```python
from build123d import *

# Parameters (mm, degrees)
SKETCH_1_R             = 7
EXTRUDE_1_DEPTH        = 160
EXTRUDE_1_DEPTH_BACK   = 36
SKETCH_2_R             = 7
EXTRUDE_2_DEPTH        = 8
SKETCH_3_W             = 18
SKETCH_3_H             = 11
EXTRUDE_3_DEPTH        = 15
EXTRUDE_4_DEPTH        = 30
SKETCH_5_W             = 60
SKETCH_5_H             = 40
EXTRUDE_5_DEPTH        = 6
SKETCH_6_W             = 60
SKETCH_6_H             = 6
EXTRUDE_6_DEPTH        = 60
SKETCH_7_W             = 29.455878384
SKETCH_7_H             = 4
EXTRUDE_7_DEPTH        = 8
PATTERN_LINEAR_1_COUNT = 2
PATTERN_LINEAR_1_PITCH = 52
SKETCH_8_W             = 118.40385017
SKETCH_8_H             = 95.184754192
CUT_EXTRUDE_1_DEPTH    = 200


with BuildPart() as part:
    # 草图1 → 凸台-拉伸1 (new body, two sides)
    with BuildSketch(Plane.XY) as extrude_1_sk:
        Circle(SKETCH_1_R)
    extrude(amount=EXTRUDE_1_DEPTH)
    extrude(extrude_1_sk.sketch, amount=-EXTRUDE_1_DEPTH_BACK)

    # 草图2 → 凸台-拉伸2 (add)
    with BuildSketch(Plane(origin=(0, 0, -36), x_dir=(-1, 0, 0), z_dir=(0, 0, -1))):
        Polygon((20, 7.5), (15, 12.5), (-15, 12.5), (-20, 7.5), (-20, -7.5), (-15, -12.5), (15, -12.5), (20, -7.5), align=None)
        Circle(SKETCH_2_R, mode=Mode.SUBTRACT)
        Circle(SKETCH_2_R)
    extrude(amount=EXTRUDE_2_DEPTH)

    # 草图3 → 凸台-拉伸3 (add)
    with BuildSketch(Plane(origin=(0, 0, -44), x_dir=(-1, 0, 0), z_dir=(0, 0, -1))):
        Rectangle(SKETCH_3_W, SKETCH_3_H)
    extrude(amount=EXTRUDE_3_DEPTH)

    # 草图4 → 凸台-拉伸4 (add)
    with BuildSketch(Plane(origin=(0, 0, -59), x_dir=(-1, 0, 0), z_dir=(0, 0, -1))):
        with BuildLine():
            Line((-15, -12.5), (-15, 12.5))
            ThreePointArc((-15, 12.5), (-27.5, 0), (-15, -12.5))
        make_face()
        with BuildLine():
            ThreePointArc((-3.77502784, 5.5), (-8.385621722, 10.606601718), (-15, 12.5))
            Line((-15, 12.5), (-15, -12.5))
            ThreePointArc((-15, -12.5), (-8.385621722, -10.606601718), (-3.77502784, -5.5))
            Line((-3.77502784, -5.5), (-9, -5.5))
            Line((-9, -5.5), (-9, 5.5))
            Line((-9, 5.5), (-3.77502784, 5.5))
        make_face()
        with BuildLine():
            ThreePointArc((-2.5, 0), (-2.822928267, 2.822928267), (-3.77502784, 5.5))
            Line((-3.77502784, 5.5), (-9, 5.5))
            Line((-9, 5.5), (-9, -5.5))
            Line((-9, -5.5), (-3.77502784, -5.5))
            ThreePointArc((-3.77502784, -5.5), (-2.822928267, -2.822928267), (-2.5, 0))
        make_face()
        with BuildLine():
            ThreePointArc((3.77502784, -5.5), (2.5, 0), (3.77502784, 5.5))
            Line((3.77502784, 5.5), (-3.77502784, 5.5))
            ThreePointArc((-3.77502784, 5.5), (-2.822928267, 2.822928267), (-2.5, 0))
            ThreePointArc((-2.5, 0), (-2.822928267, -2.822928267), (-3.77502784, -5.5))
            Line((-3.77502784, -5.5), (3.77502784, -5.5))
        make_face()
        with BuildLine():
            Line((9, 5.5), (3.77502784, 5.5))
            ThreePointArc((3.77502784, 5.5), (2.5, 0), (3.77502784, -5.5))
            Line((3.77502784, -5.5), (9, -5.5))
            Line((9, -5.5), (9, 5.5))
        make_face()
        with BuildLine():
            Line((15, -12.5), (15, 12.5))
            ThreePointArc((15, 12.5), (8.385621722, 10.606601718), (3.77502784, 5.5))
            Line((3.77502784, 5.5), (9, 5.5))
            Line((9, 5.5), (9, -5.5))
            Line((9, -5.5), (3.77502784, -5.5))
            ThreePointArc((3.77502784, -5.5), (8.385621722, -10.606601718), (15, -12.5))
        make_face()
        with BuildLine():
            ThreePointArc((27.5, 0), (23.838834765, 8.838834765), (15, 12.5))
            Line((15, 12.5), (15, -12.5))
            ThreePointArc((15, -12.5), (23.838834765, -8.838834765), (27.5, 0))
        make_face()
        with BuildLine():
            Line((-15, -12.5), (15, -12.5))
            ThreePointArc((15, -12.5), (8.385621722, -10.606601718), (3.77502784, -5.5))
            Line((3.77502784, -5.5), (-3.77502784, -5.5))
            ThreePointArc((-3.77502784, -5.5), (-8.385621722, -10.606601718), (-15, -12.5))
        make_face()
        with BuildLine():
            ThreePointArc((3.77502784, 5.5), (8.385621722, 10.606601718), (15, 12.5))
            Line((15, 12.5), (-15, 12.5))
            ThreePointArc((-15, 12.5), (-8.385621722, 10.606601718), (-3.77502784, 5.5))
            Line((-3.77502784, 5.5), (3.77502784, 5.5))
        make_face()
    extrude(amount=EXTRUDE_4_DEPTH)

    # 草图5 → 凸台-拉伸5 (add)
    with BuildSketch(Plane(origin=(0, 0, -89), x_dir=(-1, 0, 0), z_dir=(0, 0, -1))):
        Rectangle(SKETCH_5_W, SKETCH_5_H)
    extrude(amount=EXTRUDE_5_DEPTH)

    # 草图6 → 凸台-拉伸6 (add)
    with BuildSketch(Plane(origin=(0, 0, -95), x_dir=(-1, 0, 0), z_dir=(0, 0, -1))):
        with Locations((0, 17)):
            Rectangle(SKETCH_6_W, SKETCH_6_H)
        with Locations((0, -17)):
            Rectangle(SKETCH_6_W, SKETCH_6_H)
    extrude(amount=EXTRUDE_6_DEPTH)

    # 草图7 → 凸台-拉伸7 (add)
    with BuildSketch(Plane.ZY.offset(30)):
        Polygon((-125, 8), (-125, 14), (-155, 14), (-160, 14), (-160, 8), align=None)
        Polygon((-125, -8), (-160, -8), (-160, -14), (-155, -14), (-125, -14), align=None)
        Polygon((-160, 8), (-160, 14), (-166, 14), (-166, 4), (-166, 0), (-166, -4), (-166, -14), (-160, -14), (-160, -8), align=None)
        with Locations((-180.727939192, -2)):
            Rectangle(SKETCH_7_W, SKETCH_7_H)
        with Locations((-180.727939192, 2)):
            Rectangle(SKETCH_7_W, SKETCH_7_H)
    extrude_7 = extrude(amount=-EXTRUDE_7_DEPTH)

    # 阵列(线性)1: 凸台-拉伸7 ×2
    with Locations(*[(i * PATTERN_LINEAR_1_PITCH, 0, 0) for i in range(1, PATTERN_LINEAR_1_COUNT)]):
        add(extrude_7)

    # 草图8 → 切除-拉伸1 (cut)
    with BuildSketch(Plane.XY.offset(-59)):
        Rectangle(SKETCH_8_W, SKETCH_8_H)
    extrude(amount=-CUT_EXTRUDE_1_DEPTH, mode=Mode.SUBTRACT)


solid = part.part
```
Check sheet for the modelled part. Datum: model origin and axes. Units: mm. A direction names the side the tool comes from. Coordinates: 2 decimals unless noted, no trailing zeros. Write each loop counter-clockwise with the first axis right and the second up, starting at its lowest first coordinate (ties: lowest second). Pieces come first, ordered by that corner, then holes. Notation, with made-up numbers: (41, 56.25) -> (72, 56.25) arc R16 cw to (72, 83.25) -> close; hole circle Ø8 at (-10, 36). An arc over 180 degrees is marked (long way). Use a Markdown table: item, result.
1. Sectioned sample at D-D (y = -9.5). Enter the section's corners in (x, z).
Reported:
| item | result |
|---|---|
| outline | (-18, -44) -> (18, -44) -> (18, -36) -> (-18, -36) -> close |
2. Tool access check on faces 1 (the flat face through (0, -5.5, -51)), 2 (the flat face through (0, 5.5, -51)), 3 (the cylindrical face through (6.466, -2.681, 63.372)). Record the directions out of +Z, -Z, +X, -X, +Y, -Y that give a thin tool (end or side, any length) a straight path to the whole face; none if there is none.
Reported:
| item | result |
|---|---|
| face 1 | -Z, +X, -X, -Y |
| face 2 | -Z, +X, -X, +Y |
| face 3 | +Z |
3. Sectioned sample at B-B (y = 0). Enter the section's corners in (x, z).
Reported:
| item | result |
|---|---|
| outline | (-20, -44) -> (-9, -44) -> (-9, -59) -> (9, -59) -> (9, -44) -> (20, -44) -> (20, -36) -> (7, -36) -> (7, 160) -> (-7, 160) -> (-7, -36) -> (-20, -36) -> close |
4. Go/stop test with flat-tipped pins: pin 1 Ø5.5 at (y, z) = (1.5, -49) entering from -X; pin 2 Ø5 at (y, z) = (1.5, -23) entering from -X; pin 3 Ø7.5 at (x, z) = (1, -48) entering from +Y. Record where each tip stops, or that it passes through.
Reported:
| item | result |
|---|---|
| pin 1 | stops at x = -9 |
| pin 2 | stops at x = -7 |
| pin 3 | stops at y = 5.5 |
5. Sectioned sample at C-C (z = -12). Enter the section's corners in (x, y), plus the area to 3 significant figures.
Reported:
| item | result |
|---|---|
| outline | circle Ø14 at (0, 0) |
| area | 154 mm2 |
6. Sectioned sample at A-A (x = 0). Enter the section's corners in (y, z).
Reported:
| item | result |
|---|---|
| outline | (-12.5, -44) -> (-5.5, -44) -> (-5.5, -59) -> (5.5, -59) -> (5.5, -44) -> (12.5, -44) -> (12.5, -36) -> (7, -36) -> (7, 160) -> (-7, 160) -> (-7, -36) -> (-12.5, -36) -> close |
7. Scan lines: line 1 along Z through (x, y) = (1.5, -10); line 2 along Y through (x, z) = (1, -32); line 3 along Z through (x, y) = (1, 6). Record each from-to range of solid material in increasing order.
Reported:
| item | result |
|---|---|
| line 1 | z = -44 to -36 |
| line 2 | y = -6.93 to 6.93 |
| line 3 | z = -44 to 160 |
